Part model, mm, in its own coordinate system. A direction names the side the tool comes from. Give positions to 0.01 mm unless a question says otherwise; leave off trailing zeros. Write each loop counter-clockwise with the first axis right and the second up, starting at its lowest first coordinate (ties: lowest second). Pieces come first, ordered by that corner, then holes.
Autodesk Fusion 360 part; units mm, degrees
sketch "Sketch1" plane through (0, 0, 0) normal (0, 1, 0) x (1, 0, 0)
  line L0 (0, -25.4) -> (0, 0)
  line L1 (0, 0) -> (25.4, 0)
  line L2 (12.7, -12.7) -> (11.05, -11.05) construction
  line L3 (3.175, -25.4) -> (3.175, -3.175)
  line L4 (3.175, -3.175) -> (25.4, -3.175)
  line L5 (25.4, -3.175) -> (25.4, 0)
  line L6 (0, -25.4) -> (3.175, -25.4)
  dimension "d1" = 25.4
  dimension "d2" = 25.4
  dimension "d13" = 3.175
extrude "Extrude1" add sketch "Sketch1" along normal blind 300
sketch "Sketch2" plane through (3.175, 0, 0) normal (1, 0, 0) x (0, 0, -1)
  line L0 (-25.4, 0) -> (-3.175, 0)
  line L1 (-3.175, 0) -> (-3.175, 300)
  line L2 (-3.175, 300) -> (-25.4, 300)
  line L3 (-25.4, 300) -> (-25.4, 0)
  circle A0 centre (-14.2875, 287.3) radius 2.76
  circle A1 centre (-14.2875, 12.7) radius 2.5546
  line L4 (-14.2875, 300) -> (-14.2875, 0) construction
  dimension "d14" = 12.7
  dimension "d15" = 12.7
hole "Hole1" at (3.175, 12.7, 14.2875) at (3.175, 287.3, 14.2875) direction (-1, 0, 0) diameter 6.5 end through all
sketch "Sketch3" plane through (0, 0, 3.175) normal (0, 0, 1) x (1, 0, 0)
  line L0 (3.175, 0) -> (25.4, 0)
  line L1 (25.4, 0) -> (25.4, 300)
  line L2 (25.4, 300) -> (3.175, 300)
  line L3 (3.175, 300) -> (3.175, 0)
  line L4 (14.2875, 0) -> (14.2875, 300) construction
  circle A0 centre (14.2875, 285.713) radius 2.8949
  circle A1 centre (14.2875, 14.287) radius 4.0168
  dimension "d19" = 14.287
  dimension "d20" = 14.287
hole "Hole2" at (14.2875, 14.287, 3.175) at (14.2875, 285.713, 3.175) direction (0, 0, -1) diameter 6.5 end through all
equation "d14 = ( 25.4 / 2 ) * 1 mm"
equation "d15 = ( 25.4 / 2 ) * 1 mm"
equation "d19 = 25.4 mm - 11.113 mm"
1) Drill centre lines: L1, parallel to Z at x = 2, y = 287.3; L2, parallel to X at y = 58.5, z = 24 (3 decimals). Where is each one in solid material? Low to high.
Check result:
L1: z = 0 to 11.04, 17.54 to 25.4
L2: x = 0 to 3.175
2) Mould opens along X. For faces 1 (the flat face through (0, 148, 13)), 2 (the flat face through (13, 148, 0)), 3 (the cylindrical face through (16.265, 16.866, 1.565)) say: +X half, -X half, draft (parallel to the pull), parting line (faces both ways), or undercut.
Check result:
face 1: -X half
face 2: draft
face 3: undercut
3) Saw through at A-A (y = 221). Write the cut outline in (x, z) (3 decimals), and give its area (3 significant figures).
Check result:
outline: (0, 0) - (25.4, 0) - (25.4, 3.175) - (3.175, 3.175) - (3.175, 25.4) - (0, 25.4) - close
area: 151 mm2
4) 3-axis set-ups, long thin cutter, end or side, ignore diameter. For faces 4 (the flat face through (3.175, 148, 14)), 5 (the cylindrical face through (1.57, 10.5, 16.68)): which of +Z, -Z, +X, -X, +Y, -Y reach the whole face in a straight line?
Check result:
face 4: +Z, +X, +Y, -Y
face 5: +X, -X
5) Flat gauge pin, fed straight in: P1, Ø7.5, axis at x = 14.29, y = 14.29, coming from the +Z side (3 decimals). Where does the tip first touch, or does it go through?
Check result:
P1: stops at z = 3.175
6) Saw through at B-B (z = 21). Write the cut outline in (x, y) (3 decimals).
Check result:
outline: (0, 0) - (3.175, 0) - (3.175, 300) - (0, 300) - close
7) Saw through at C-C (x = 6.75). Write the cut outline in (y, z) (3 decimals).
Check result:
outline: (0, 0) - (300, 0) - (300, 3.175) - (0, 3.175) - close
